```python
from build123d import *

# Parameters (mm, degrees)
SKETCH_1_W                = 60
SKETCH_1_H                = 50
EXTRUDE_1_DEPTH           = 10
HOLE_WIZARD_1_D           = 8.5
HOLE_WIZARD_1_DEPTH       = 20
HOLE_WIZARD_2_D           = 8
HOLE_WIZARD_2_CSINK_D     = 8.2
HOLE_WIZARD_2_CSINK_ANGLE = 45
HOLE_WIZARD_3_D           = 5.2


with BuildPart() as part:
    # 草图1 → 凸台-拉伸1 (new body)
    with BuildSketch(Plane.XY):
        Rectangle(SKETCH_1_W, SKETCH_1_H)
    extrude(amount=EXTRUDE_1_DEPTH)

    # 孔1
    with Locations(Plane.XY.offset(10)):
        with Locations((0, 0)):
            Hole(HOLE_WIZARD_1_D / 2, depth=HOLE_WIZARD_1_DEPTH)

    # 孔2 (through all)
    with Locations(Plane.XY.offset(10)):
        with Locations((20, 0), (-20, 0)):
            CounterSinkHole(HOLE_WIZARD_2_D / 2, HOLE_WIZARD_2_CSINK_D / 2, counter_sink_angle=HOLE_WIZARD_2_CSINK_ANGLE)

    # 孔3 (through all)
    with Locations(Plane(origin=(0, 0, 0), x_dir=(-1, 0, 0), z_dir=(0, 0, -1))):
        with Locations((0, 18), (0, -18)):
            Hole(HOLE_WIZARD_3_D / 2)


solid = part.part
```
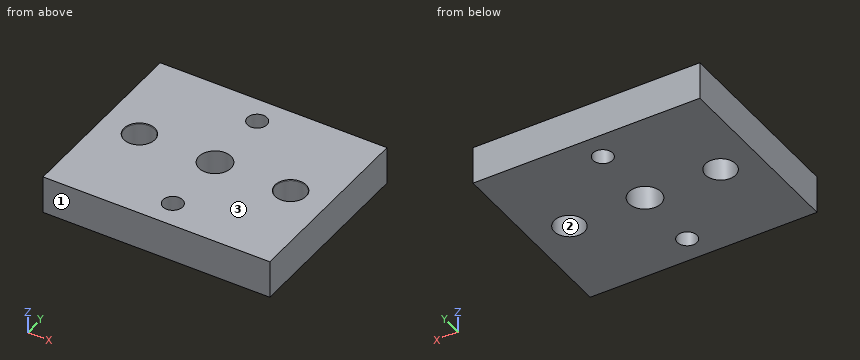
For this review, take the finished solid that the model builds, in its own axes (mm). Face numbers are marked on the shaded views. Coordinates: 2 decimals unless noted, no trailing zeros. Loops run counter-clockwise (first coordinate to the right, second up) from the corner with the lowest first, then second, coordinate; pieces in that order, holes last.
1. Add section A-A, the plane y = 0. Give the boundary of the cut face in (x, z).
2. Mouldability with a two-part tool opening along Y and no side actions: class the marked faces 1, 2 and 3 as +Y half, -Y half, draft (parallel to the pull), parting line (faces both ways), or undercut.
3. For line 1 (Y direction, x = 0, z = 7); line 2 (X direction, y = -2, z = 3.5); line 3 (Y direction, x = 2, z = 3.75), list the stretches that pass through material, from the lowest coordinate up.
4. Add section C-C, the plane y = -18. Give the boundary of the cut face in (x, z), then the cut area to 3 significant figures.
5. Add section B-B, the plane x = 0. Give the boundary of the cut face in (y, z), then the cut area to 3 significant figures.
6. Add section D-D, the plane z = 5.5. Give the boundary of the cut face in (x, y), then the cut area to 3 significant figures.
Result:
1. outline: (-30, 0) - (-24, 0) - (-24, 9.76) - (-24.1, 10) - (-30, 10) - close; (-16, 0) - (-4.25, 0) - (-4.25, 10) - (-15.9, 10) - (-16, 9.76) - close; (4.25, 0) - (16, 0) - (16, 9.76) - (15.9, 10) - (4.25, 10) - close; (24, 0) - (30, 0) - (30, 10) - (24.1, 10) - (24, 9.76) - close
2. face 1: -Y half
2. face 2: undercut
2. face 3: draft
3. line 1: y = -25 to -20.6, -15.4 to -4.25, 4.25 to 15.4, 20.6 to 25
3. line 2: x = -30 to -23.46, -16.54 to -3.75, 3.75 to 16.54, 23.46 to 30
3. line 3: y = -25 to -19.66, -16.34 to -3.75, 3.75 to 16.34, 19.66 to 25
4. outline: (-30, 0) - (-2.6, 0) - (-2.6, 10) - (-30, 10) - close; (2.6, 0) - (30, 0) - (30, 10) - (2.6, 10) - close
4. area: 548 mm2
5. outline: (-25, 0) - (-20.6, 0) - (-20.6, 10) - (-25, 10) - close; (-15.4, 0) - (-4.25, 0) - (-4.25, 10) - (-15.4, 10) - close; (4.25, 0) - (15.4, 0) - (15.4, 10) - (4.25, 10) - close; (20.6, 0) - (25, 0) - (25, 10) - (20.6, 10) - close
5. area: 311 mm2
6. outline: (-30, -25) - (30, -25) - (30, 25) - (-30, 25) - close; hole circle Ø8 at (-20, 0); hole circle Ø8.5 at (0, 0); hole circle Ø5.2 at (0, -18); hole circle Ø5.2 at (0, 18); hole circle Ø8 at (20, 0)
6. area: 2,800 mm2
